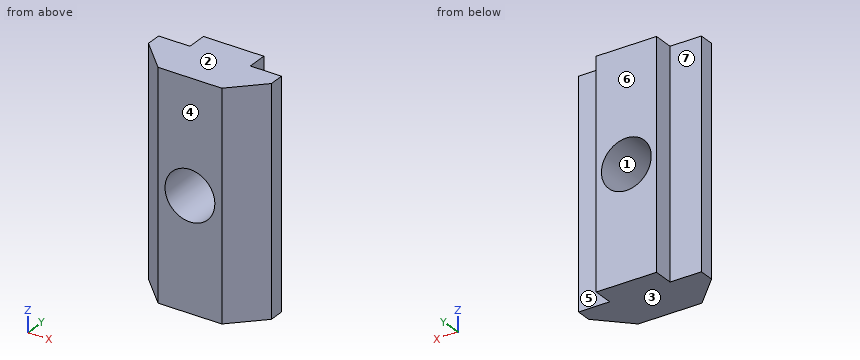
Autodesk Inventor part; units mm, degrees
ref_plane "YZ Plane" through (0, 0, 0) normal (1, 0, 0) x (0, 1, 0)
ref_plane "XZ Plane" through (0, 0, 0) normal (0, 1, 0) x (-1, 0, 0)
ref_plane "XY Plane" through (0, 0, 0) normal (0, 0, 1) x (1, 0, 0)
sketch "Boceto1" plane through (0, 0, 0) normal (0, 0, 1) x (1, 0, 0)
  line L0 (0, 0) -> (-2.65, 2.65)
  line L1 (8.35, 2.65) -> (5.7, 0)
  line L2 (8.35, 4) -> (8.35, 2.65)
  line L3 (-2.65, 4) -> (8.35, 4)
  line L4 (-2.65, 2.65) -> (-2.65, 4)
  line L5 (5.7, 0) -> (0, 0)
  dimension "d1" = 11
  dimension "d2" = 5.7
  dimension "d5" = 2.65
  dimension "d6" = 2.65
  dimension "d7" = 4
  dimension "d9" = 45
  dimension "d10" = 45
extrude "Extrusión1" add sketch "Boceto1" along normal blind 20
sketch "Boceto3" plane through (-2.65, 4, 0) normal (0, 1, 0) x (1, 0, 0)
  line L0 (11, 0) -> (0, 0)
  line L1 (8.2, 0) -> (2.8, 0)
  line L2 (2.8, 0) -> (2.8, -20)
  line L3 (2.8, -20) -> (8.2, -20)
  line L4 (8.2, -20) -> (8.2, 0)
  line L5 (11, -20) -> (0, -20)
  line L6 (11, 0) -> (11, -20)
  line L7 (0, 0) -> (0, -20)
  point P0 (2.65, 0)
  point P1 (5.5, -20)
  point P2 (2.8, 0)
  dimension "d20" = 2.8
  dimension "d21" = 2.8
extrude "Extrusión2" add sketch "Boceto3" along normal blind 1.8 contours L4 L3 L2 L0
sketch "Boceto4" plane through (-2.65, 5.8, 0) normal (0, 1, 0) x (1, 0, 0)
  line L0 (8.2, 0) -> (2.8, 0)
  line L1 (5.5, 0) -> (5.5, -20)
  line L2 (2.8, -20) -> (8.2, -20)
  line L3 (2.8, 0) -> (2.8, -20)
  line L4 (2.8, -10) -> (5.5, -10)
  point P0 (2.65, 0)
hole "Agujero2" at (2.85, 5.8, 10) direction (0, -1, 0) diameter 4.4587 depth 10
properties part number "Pasador" material "Aluminio 6061"
Verification items for the finished model (mm, model axes). Face numbers are marked on the shaded views. A direction names the side the tool comes from. Give positions to 0.01 mm unless a question says otherwise; leave off trailing zeros. Order: outer loops, then holes, each group sorted by start corner. A loop starts at its lowest first (then second) coordinate and runs counter-clockwise, first axis right, second up. Notation, with made-up numbers: M 81,22.5 L 99,22.5 A24 cw 99,45.5 Z; hole C 25.5,6 d10. An arc over 180 degrees is marked long. Answer in a Markdown table with one row per item. Add a question column.
Item 1: Section check D-D, the plane z = 16. Enter the section's corners in (x, y), and give its area (3 significant figures).
Item 2: Scan lines: probe 1 along Z at (x, y) = (2.85, 4.4); probe 2 along X at (y, z) = (2.75, 10); probe 3 along X at (y, z) = (4.6, 10). Record each from-to range of solid material in increasing order. Write a range as from..to.
Item 3: Section check C-C, the plane y = 0.8. Enter the section's corners in (x, z), and give its area (3 significant figures).
Item 4: Tool access check on the marked faces 5, 6 and 7. Record the directions out of +Z, -Z, +X, -X, +Y, -Y that give a thin tool (end or side, any length) a straight path to the whole face; none if there is none.
Item 5: Section check A-A, the plane x = 2.85. Enter the section's corners in (y, z), and give its area (3 significant figures).
Item 6: Section check B-B, the plane z = 10. Enter the section's corners in (x, y).
Item 7: Mould release check, pull along Z, two halves, no side actions. Record for the marked faces 1, 2, 3 and 4: released by +Z, released by -Z, zero draft, split by the parting line, or undercut.
Item 8: Gauge pin test, flat ends, axial feed: pin 1 (0.8 mm diameter, centred on x = -2, z = 6.5, fed in from +Y); pin 2 (0.5 mm diameter, centred on y = 5.5, z = 11, fed in from +X); pin 3 (0.5 mm diameter, centred on y = 4.5, z = 14.5, fed in from -X). Record the tip position at first contact, or that the pin passes through.
Filled sheet:
| question | item | result |
|---|---|---|
| 1 | outline | M -2.65,2.65 L 0,0 L 5.7,0 L 8.35,2.65 L 8.35,4 L 5.55,4 L 5.55,5.8 L 0.15,5.8 L 0.15,4 L -2.65,4 Z |
| 1 | area | 46.7 mm^2 |
| 2 | probe 1 | z = 0..7.77, 12.23..20 |
| 2 | probe 2 | x = -2.65..0.62, 5.08..8.35 |
| 2 | probe 3 | x = 0.15..0.62, 5.08..5.55 |
| 3 | outline | M -0.8,0 L 6.5,0 L 6.5,20 L -0.8,20 Z; hole C 2.85,10 d4.46 |
| 3 | area | 130 mm^2 |
| 4 | face 5 | +Z, -Z, +X, +Y |
| 4 | face 6 | +Z, -Z, +X, -X, +Y |
| 4 | face 7 | +Z, -Z, -X, +Y |
| 5 | outline | M 0,0 L 5.8,0 L 5.8,7.77 L 0,7.77 Z; M 0,12.23 L 5.8,12.23 L 5.8,20 L 0,20 Z |
| 5 | area | 90.1 mm^2 |
| 6 | outline | M -2.65,2.65 L 0,0 L 0.62,0 L 0.62,5.8 L 0.15,5.8 L 0.15,4 L -2.65,4 Z; M 5.08,0 L 5.7,0 L 8.35,2.65 L 8.35,4 L 5.55,4 L 5.55,5.8 L 5.08,5.8 Z |
| 7 | face 1 | undercut |
| 7 | face 2 | released by +Z |
| 7 | face 3 | released by -Z |
| 7 | face 4 | zero draft |
| 8 | pin 1 | stops at y = 4 |
| 8 | pin 2 | stops at x = 5.55 |
| 8 | pin 3 | stops at x = 0.15 |
